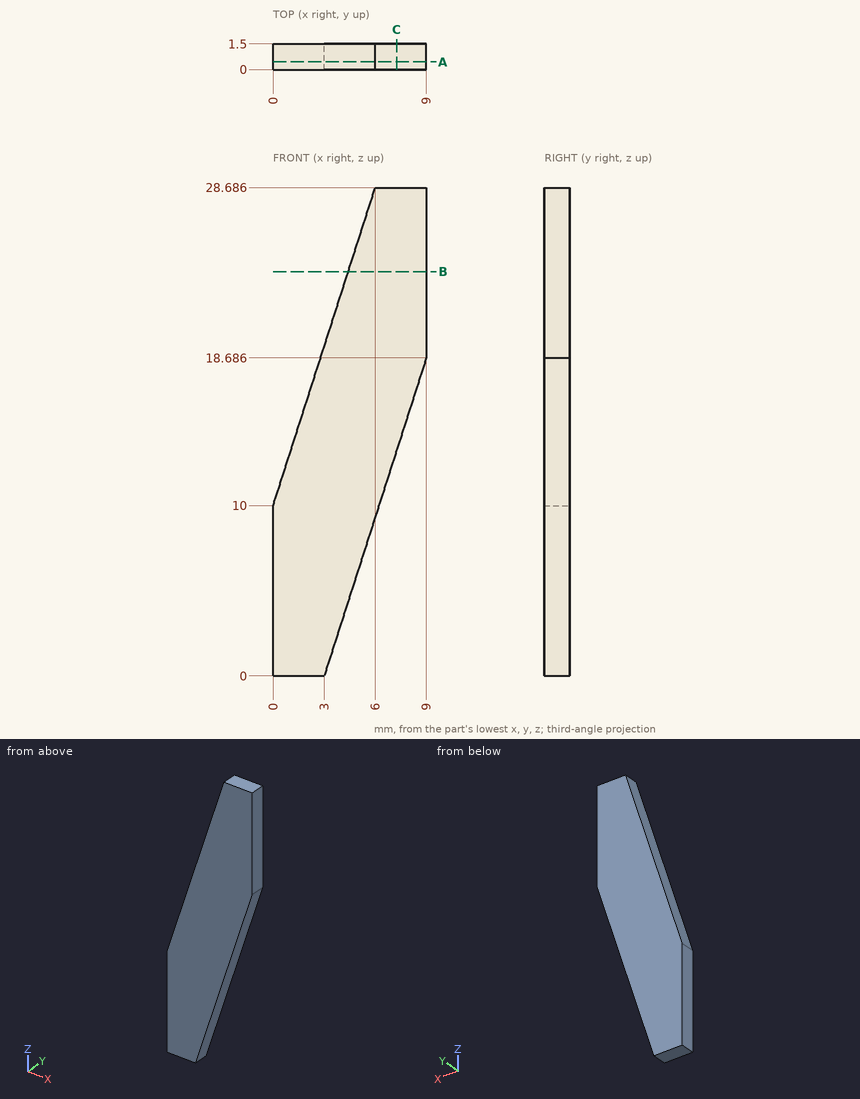
Check sheet for the drawn part. Datum: minimum x, y, z corner. Units: mm. Round coordinates to 2 decimals unless told otherwise and drop trailing zeros. Loops run counter-clockwise (first coordinate to the right, second up) from the corner with the lowest first, then second, coordinate; pieces in that order, holes last. Notation, with made-up numbers: M 82.5,-14 L 89.5,-14 A25 ccw 89.5,2 Z; hole C 27.5,40.25 d9. An arc over 180 degrees is marked long. One line per question, with ' | ' between items. Start each with the question number.
Item 1: Section check C-C (x = 7.25). Record the boundary of the cut face in (y, z), and give its area (3 significant figures).
Item 2: Scan lines: probe 1 along X at (y, z) = (0.2, 6.25); probe 2 along X at (y, z) = (1.2, 1). Record each from-to range of solid material in increasing order.
Item 3: Section check B-B (z = 23.75). Record the boundary of the cut face in (x, y) (1 decimal).
Item 4: Section check A-A (y = 0.45). Record the boundary of the cut face in (x, z), and give its area (3 significant figures).
Worked out:
1) outline: M 0,13.24 L 1.5,13.24 L 1.5,28.69 L 0,28.69 Z | area: 23.2 mm^2
2) probe 1: 0 to 5.01 | probe 2: 0 to 3.32
3) outline: M 4.4,0 L 9,0 L 9,1.5 L 4.4,1.5 Z
4) outline: M 0,0 L 3,0 L 9,18.69 L 9,28.69 L 6,28.69 L 0,10 Z | area: 146 mm^2
